The model under review builds one solid part; all positions refer to its coordinate system, in mm. Face numbers are marked on the shaded views. A direction names the side the tool comes from. Round coordinates to 2 decimals unless told otherwise and drop trailing zeros. Order: outer loops, then holes, each group sorted by start corner. A loop starts at its lowest first (then second) coordinate and runs counter-clockwise, first axis right, second up. Notation, with made-up numbers: (73, 31) - (106, 31) arc R20 cw to (106, 36) - close; hole circle Ø4 at (64.5, -21.75). An arc over 180 degrees is marked (long way). One line per question, with ' | ' between items. Start each with the question number.
Item 1: Tool access review of the marked faces 1 and 2: name each direction out of +Z, -Z, +X, -X, +Y, -Y from which nothing blocks a thin tool from reaching the whole face with its end or side.
Item 2: Add section B-B on x = 0. State the section outline as (y, z) points, and give its area (3 significant figures).
Item 3: For L1, parallel to Y at x = 0.25, z = -4; L2, parallel to X at y = 1.1, z = -0.5; L3, parallel to Z at x = -2, y = 0.6, list the stretches that pass through material, from the lowest coordinate up. Write a range as [from, to].
Item 4: Add section A-A on z = 0. State the section outline as (x, y) points, and give its area (3 significant figures).
Item 5: Add section C-C on y = 1.6. State the section outline as (x, z) points, and give its area (3 significant figures).
Item 6: Add section D-D on z = -3.75. State the section outline as (x, y) points.
Item 7: Insertion check: pin 1 Ø1.5 at (x, y) = (-3.5, 2) entering from +Z. The pin has a flat end and moves straight along its axis. Give the tip position at first contact, or say it passes through.
Autodesk Inventor part; units mm, degrees
sketch "Sketch1" plane through (0, 0, 0) normal (0, 1, 0) x (-1, 0, 0)
  line L0 (5, -5) -> (-5, -5)
  line L1 (-5, -5) -> (-5, 5)
  line L2 (-5, 5) -> (5, 5)
  line L3 (5, 5) -> (5, -5)
  line L4 (0, -6.825) -> (0, 6.825)
  line L5 (-7, 0) -> (7, 0)
  point P0 (0, 0)
  point P1 (0, -5)
  point P2 (5, 0)
  dimension "d0" = 10
  dimension "d1" = 10
extrude "Extrusion1" add sketch "Sketch1" along normal mid plane 1
sketch "Sketch2" plane through (0, 0.5, 0) normal (0, 1, 0) x (1, 0, 0)
  circle A0 centre (0, 0) radius 2.5
  dimension "d4" = 5
extrude "Extrusion2" add sketch "Sketch2" along normal blind 2.5
properties part number "1x1_Piece"
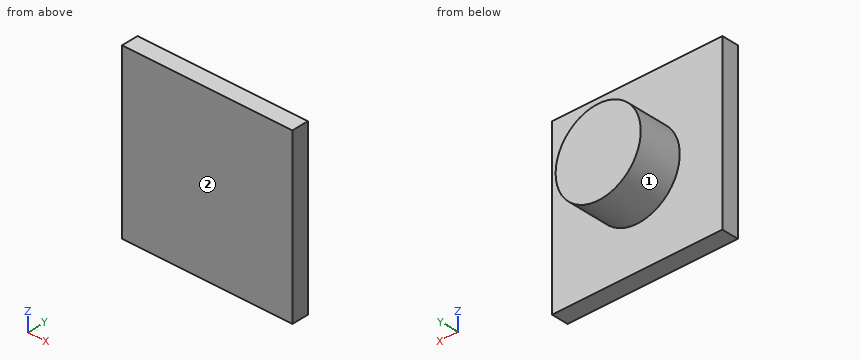
Determined:
1) face 1: +Y | face 2: +Z, -Z, +X, -X, -Y
2) outline: (-0.5, -5) - (0.5, -5) - (0.5, -2.5) - (3, -2.5) - (3, 2.5) - (0.5, 2.5) - (0.5, 5) - (-0.5, 5) - close | area: 22.5 mm2
3) L1: [-0.5, 0.5] | L2: [-2.45, 2.45] | L3: [-1.5, 1.5]
4) outline: (-5, -0.5) - (5, -0.5) - (5, 0.5) - (2.5, 0.5) - (2.5, 3) - (-2.5, 3) - (-2.5, 0.5) - (-5, 0.5) - close | area: 22.5 mm2
5) outline: circle Ø5 at (0, 0) | area: 19.6 mm2
6) outline: (-5, -0.5) - (5, -0.5) - (5, 0.5) - (-5, 0.5) - close
7) pin 1: through
